Part model, mm, in its own coordinate system. Round coordinates to 2 decimals unless told otherwise and drop trailing zeros. Loops run counter-clockwise (first coordinate to the right, second up) from the corner with the lowest first, then second, coordinate; pieces in that order, holes last. Notation, with made-up numbers: M 15.5,26 L 37.5,26 A18 ccw 37.5,38 Z; hole C 3.25,-17.75 d4. An arc over 180 degrees is marked long. Put each result on its own line as item: value. Start each with the question number.
```python
from build123d import *

# Parameters (mm, degrees)
SKETCH1_W           = 50
SKETCH1_H           = 350
SKETCH1_H_2         = 50
SKETCH1_W_2         = 350
BOSS_EXTRUDE1_DEPTH = 20
FILLET1_R           = 10
SKETCH2_R           = 5
CUT_EXTRUDE1_DEPTH  = 20


with BuildPart() as part:
    # Sketch1 → Boss-Extrude1 (new body)
    with BuildSketch(Plane.XY):
        with Locations((25, 175)):
            Rectangle(SKETCH1_W, SKETCH1_H)
        with Locations((25, 375)):
            Rectangle(SKETCH1_W, SKETCH1_H_2)
        with Locations((225, 375)):
            Rectangle(SKETCH1_W_2, SKETCH1_H_2)
    extrude(amount=BOSS_EXTRUDE1_DEPTH)

    # Fillet1
    fillet1_edges = [part.edges().sort_by_distance(p)[0] for p in [
        (50, 0, 10),
        (0, 0, 10),
        (0, 400, 10),
        (400, 400, 10),
        (400, 350, 10),
        (50, 350, 10),
    ]]
    fillet(fillet1_edges, radius=FILLET1_R)

    # Sketch2 → Cut-Extrude1 (cut)
    with BuildSketch(Plane.XY.offset(20)):
        with Locations((25, 30)):
            Circle(SKETCH2_R)
        with Locations((30, 370)):
            Circle(SKETCH2_R)
        with Locations((370, 375)):
            Circle(SKETCH2_R)
    extrude(amount=-CUT_EXTRUDE1_DEPTH, mode=Mode.SUBTRACT)


solid = part.part
```
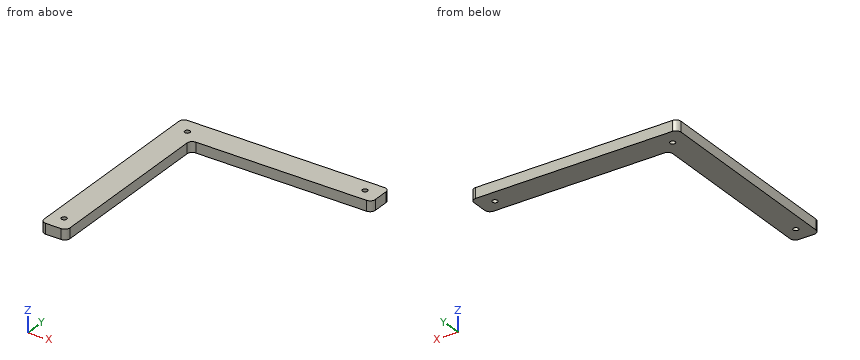
1. Cut at B-B, the plane y = 30. Give the cut face in (x, z), and give its area (3 significant figures).
2. Wall check: L1, parallel to Y at x = 371, z = 3.25; L2, parallel to X at y = 29, z = 5.5; L3, parallel to X at y = 132, z = 9.5. Give the ranges that are in metal, low to high.
3. Cut at D-D, the plane y = 98. Give the cut face in (x, z), and give its area (3 significant figures).
4. Cut at C-C, the plane z = 5.5. Give the cut face in (x, y).
5. Drop flat-ended pins along their axis: pin 1 (1.5 mm diameter, centred on x = 222.5, z = 13.5, fed in from -Y); pin 2 (5 mm diameter, centred on y = 140.5, z = 5.5, fed in from +X). Give the stop position or say it passes through.
6. Cut at A-A, the plane x = 370. Give the cut face in (y, z).
Results list:
1. outline: M 0,0 L 20,0 L 20,20 L 0,20 Z; M 30,0 L 50,0 L 50,20 L 30,20 Z
1. area: 800 mm^2
2. L1: y = 350 to 370.1, 379.9 to 400
2. L2: x = 0 to 20.1, 29.9 to 50
2. L3: x = 0 to 50
3. outline: M 0,0 L 50,0 L 50,20 L 0,20 Z
3. area: 1,000 mm^2
4. outline: M 0,10 A10 ccw 10,0 L 40,0 A10 ccw 50,10 L 50,340 A10 cw 60,350 L 390,350 A10 ccw 400,360 L 400,390 A10 ccw 390,400 L 10,400 A10 ccw 0,390 Z; hole C 25,30 d10; hole C 30,370 d10; hole C 370,375 d10
5. pin 1: stops at y = 350
5. pin 2: stops at x = 50
6. outline: M 350,0 L 370,0 L 370,20 L 350,20 Z; M 380,0 L 400,0 L 400,20 L 380,20 Z
